from build123d import *

# Parameters (mm, degrees)
SKETCH_1_R          = 30
SKETCH_1_R_2        = 13.5
SKETCH_1_R_3        = 1.880556804
EXTRUDE_1_DEPTH     = 10
SKETCH_2_W          = 60
SKETCH_2_H          = 5
EXTRUDE_2_DEPTH     = 60
CUT_EXTRUDE_START   = -5
SKETCH_7_R          = 30
CUT_EXTRUDE_4_DEPTH = 5


with BuildPart() as part:
    # 草图1 → 凸台-拉伸1 (new body)
    # profile 1 of 5: a face of its own
    with BuildSketch(Plane.XY):
        Circle(SKETCH_1_R)
        Circle(SKETCH_1_R_2, mode=Mode.SUBTRACT)
    # profile 2 of 5: a face of its own
    with BuildSketch(Plane.XY):
        Circle(SKETCH_1_R_2)
    # profile 3 of 5: a face of its own
    with BuildSketch(Plane.XY):
        with Locations((0, 13.5)):
            Circle(SKETCH_1_R_3)
    # profile 4 of 5: a face of its own
    with BuildSketch(Plane.XY):
        with Locations((-11.691342951, -6.75)):
            Circle(SKETCH_1_R_3)
    # profile 5 of 5: a face of its own
    with BuildSketch(Plane.XY):
        with Locations((11.691342951, -6.75)):
            Circle(SKETCH_1_R_3)
    extrude(amount=EXTRUDE_1_DEPTH)

    # 草图2 → 凸台-拉伸2 (add)
    with BuildSketch(Plane(origin=(0, 0, 0), x_dir=(-1, 0, 0), z_dir=(0, 0, -1))):
        Rectangle(SKETCH_2_W, SKETCH_2_H)
    extrude(amount=EXTRUDE_2_DEPTH)

    # 草图7 → 切除-拉伸4 (cut)
    with BuildSketch(Plane.XY.offset(10).offset(CUT_EXTRUDE_START)):
        Circle(SKETCH_7_R)
    extrude(amount=CUT_EXTRUDE_4_DEPTH, mode=Mode.SUBTRACT)


solid = part.part
Read the model definition and answer for the solid it produces. Units are mm, in the model's axes. A direction names the side the tool comes from. Give positions to 0.01 mm unless a question says otherwise; leave off trailing zeros. Loops run counter-clockwise (first coordinate to the right, second up) from the corner with the lowest first, then second, coordinate; pieces in that order, holes last. Notation, with made-up numbers: (69, 85.25) -> (120, 85.25) arc R16 cw to (120, 106.25) -> close; hole circle Ø4 at (67.25, 53.25). An arc over 180 degrees is marked (long way). Use a Markdown table: item, result.
Q1. Find the intervals of material crossed by line 1 along Y through (x, z) = (-18.5, -53.5); line 2 along Z through (x, y) = (-14.5, 25.5), in increasing order.
Solved:
| item | result |
|---|---|
| line 1 | y = -2.5 to 2.5 |
| line 2 | z = 0 to 5 |
Q2. Section D-D, the plane x = -23 is taken. Determine the outline of the cut face in (y, z), then the cut area to 3 significant figures.
Solved:
| item | result |
|---|---|
| outline | (-19.26, 0) -> (-2.5, 0) -> (-2.5, -60) -> (2.5, -60) -> (2.5, 0) -> (19.26, 0) -> (19.26, 5) -> (-19.26, 5) -> close |
| area | 493 mm^2 |
Q3. Section A-A, the plane x = 0 is taken. Determine the outline of the cut face in (y, z).
Solved:
| item | result |
|---|---|
| outline | (-30, 0) -> (-2.5, 0) -> (-2.5, -60) -> (2.5, -60) -> (2.5, 0) -> (30, 0) -> (30, 5) -> (-30, 5) -> close |
Q4. Each of these flat-tipped pins is pushed along its axis until it touches: pin 1 (18 mm diameter, centred on x = -3.5, z = -29, fed in from -Y); pin 2 (8.5 mm diameter, centred on x = -6.5, y = -23, fed in from -Z); pin 3 (5 mm diameter, centred on x = -20, z = -19.5, fed in from +Y). Where does it stop, or does it pass through?
Solved:
| item | result |
|---|---|
| pin 1 | stops at y = -2.5 |
| pin 2 | stops at z = 0 |
| pin 3 | stops at y = 2.5 |
Q5. Section B-B, the plane z = -31 is taken. Determine the outline of the cut face in (x, y), then the cut area to 3 significant figures.
Solved:
| item | result |
|---|---|
| outline | (-30, -2.5) -> (30, -2.5) -> (30, 2.5) -> (-30, 2.5) -> close |
| area | 300 mm^2 |
Q6. Section C-C, the plane y = 14.5 is taken. Determine the outline of the cut face in (x, z).
Solved:
| item | result |
|---|---|
| outline | (-26.26, 0) -> (26.26, 0) -> (26.26, 5) -> (-26.26, 5) -> close |
Q7. A tool of negligible diameter and unlimited length cuts with its end or side. For faces 1 (the face through (0, -2.5, -30)), 2 (the face through (0, 13, 0)), 3 (the face through (30, 0, -30)), from which of +Z, -Z, +X, -X, +Y, -Y can it reach the whole face along a straight path? Write none if from no direction.
Solved:
| item | result |
|---|---|
| face 1 | -Z, +X, -X, -Y |
| face 2 | -Z, +X, -X, +Y |
| face 3 | +Z, -Z, +X, +Y, -Y |
